from build123d import *

# Parameters (mm, degrees)
F0_W      = 35
F0_H      = 35
F1_DEPTH  = 40
F2_R      = 2.5
F3_DEPTH  = 20
F5_DEPTH  = 4.4
F6_R      = 4.25
F7_DEPTH  = 21
F8_R      = 2.5
F9_DEPTH  = 14.6
F11_DEPTH = 1.9
F12_R     = 0.5
F13_DEPTH = 4


with BuildPart() as f1:
    # F0 (on Top) → F1 (new body)
    with BuildSketch(Plane.XY):
        Rectangle(F0_W, F0_H)
    extrude(amount=F1_DEPTH)

    # F2 (on face) → F3 (cut)
    with BuildSketch(Plane(origin=(0, 0, 0), x_dir=(1, 0, 0), z_dir=(0, 0, -1))):
        with Locations((-10, 0)):
            Circle(F2_R)
        with Locations((10, 0)):
            Circle(F2_R)
    extrude(amount=-F3_DEPTH, mode=Mode.SUBTRACT)

    # F4 (on face) → F5 (cut)
    with BuildSketch(Plane.XY.offset(40)):
        Polygon((-17.5, -17.5), (17.5, -17.5), (17.5, -2.5), (3.35, -2.5), (3.35, 17.5), (-3.35, 17.5), (-3.35, -2.5), (-17.5, -2.5), align=None)
    extrude(amount=-F5_DEPTH, mode=Mode.SUBTRACT)

    # F6 (on face) → F7 (cut)
    with BuildSketch(Plane(origin=(0, 0, 0), x_dir=(1, 0, 0), z_dir=(0, 0, -1))):
        with Locations((0, -5.05)):
            Circle(F6_R)
    extrude(amount=-F7_DEPTH, mode=Mode.SUBTRACT)

    # F8 (on face) → F9 (cut, through all)
    with BuildSketch(Plane(origin=(0, 0, 21), x_dir=(1, 0, 0), z_dir=(0, 0, -1))):
        with Locations((0, -5.05)):
            Circle(F8_R)
    extrude(amount=-F9_DEPTH, mode=Mode.SUBTRACT)

    # F10 (on face) → F11 (cut)
    with BuildSketch(Plane.XY.offset(35.6)):
        Polygon((-5, -17.5), (5, -17.5), (5, -10.5), (1.575, -10.5), (1.575, -2.65), (-1.575, -2.65), (-1.575, -10.5), (-5, -10.5), align=None)
    extrude(amount=-F11_DEPTH, mode=Mode.SUBTRACT)

    # F12 (on face) → F13 (cut)
    with BuildSketch(Plane.XY.offset(35.6)):
        with Locations((-2.025, -9)):
            Circle(F12_R)
        with Locations((-2.025, -4)):
            Circle(F12_R)
        with Locations((2.025, -9)):
            Circle(F12_R)
        with Locations((2.025, -4)):
            Circle(F12_R)
        with Locations((-0.975, -2.2)):
            Circle(F12_R)
        with Locations((0.975, -2.2)):
            Circle(F12_R)
    extrude(amount=-F13_DEPTH, mode=Mode.SUBTRACT)


solid = f1.part
CAD build for the part. Positions are in the model's coordinates, mm. A direction names the side the tool comes from. Give positions to 0.01 mm unless a question says otherwise; leave off trailing zeros. Write each loop counter-clockwise with the first axis right and the second up, starting at its lowest first coordinate (ties: lowest second). Pieces come first, ordered by that corner, then holes. Notation, with made-up numbers: M 13,68 L 52,68 A26 cw 52,106 Z; hole C 21,69.25 d5. An arc over 180 degrees is marked long. Put each result on its own line as item: value. Start each with the question number.
(1) Band-saw the part on D-D, the plane y = 5.05. Write the cut outline in (x, z), and give its area (3 significant figures).
(2) Band-saw the part on B-B, the plane z = 35. Write the cut outline in (x, y) (3 decimals).
(3) Band-saw the part on C-C, the plane x = -10. Write the cut outline in (y, z), and give its area (3 significant figures).
(4) Which spindle directions (+Z, -Z, +X, -X, +Y, -Y) get a long thin tool onto all of the face, cutting with end or side? Do faces 4 (the face through (10, 0, 20)), 5 (the face through (1.575, -3, 35)), 6 (the face through (-2.525, -3.978, 33.628)), 7 (the face through (3.35, 7, 38)), 8 (the face through (0, 0, 0)). Say none if no direction does.
(5) Band-saw the part on A-A, the plane y = -13. Write the cut outline in (x, z).
(6) Mould opens along Y. For faces 1 (the face through (10, 8, 40)), 2 (the face through (3, -10.5, 35)), 3 (the face through (2, -4, 31.6)) say: +Y half, -Y half, draft (parallel to the pull), parting line (faces both ways), or undercut.
(7) Flat gauge pins, fed straight in: pin 1 Ø1.1 at (x, y) = (2, -9) entering from +Z; pin 2 Ø3.5 at (x, z) = (-9, 37.5) entering from -Y; pin 3 Ø4 at (x, y) = (-10, 0) entering from -Z; pin 4 Ø4 at (x, y) = (13, 4) entering from -Z. Where does each tip first touch, or does it go through?
(8) Probe L1, parallel to X at y = 0, z = 15; L2, parallel to X at y = 5.05, z = 27. List the from-to ranges inside material, lowest first.
Response values:
1. outline: M -17.5,0 L -4.25,0 L -4.25,21 L -2.5,21 L -2.5,35.6 L -3.35,35.6 L -3.35,40 L -17.5,40 Z; M 2.5,21 L 4.25,21 L 4.25,0 L 17.5,0 L 17.5,40 L 3.35,40 L 3.35,35.6 L 2.5,35.6 Z
1. area: 1,120 mm2
2. outline: M -17.5,-17.5 L -5,-17.5 L -5,-10.5 L -1.575,-10.5 L -1.575,-9.218 A0.5 cw long -1.575,-8.782 L -1.575,-4.218 A0.5 cw long -1.575,-3.782 L -1.575,-2.65 L -1.193,-2.65 A0.5 cw long -0.757,-2.65 L 0.757,-2.65 A0.5 cw long 1.193,-2.65 L 1.575,-2.65 L 1.575,-3.782 A0.5 cw long 1.575,-4.218 L 1.575,-8.782 A0.5 cw long 1.575,-9.218 L 1.575,-10.5 L 5,-10.5 L 5,-17.5 L 17.5,-17.5 L 17.5,17.5 L -17.5,17.5 Z; hole C 0,5.05 d5
3. outline: M -17.5,0 L -2.5,0 L -2.5,20 L 2.5,20 L 2.5,0 L 17.5,0 L 17.5,40 L -2.5,40 L -2.5,35.6 L -17.5,35.6 Z
3. area: 1,230 mm2
4. face 4: -Z
4. face 5: +Z, -Y
4. face 6: +Z
4. face 7: +Z, +Y, -Y
4. face 8: -Z, +X, -X, +Y, -Y
5. outline: M -17.5,0 L 17.5,0 L 17.5,35.6 L 5,35.6 L 5,33.7 L -5,33.7 L -5,35.6 L -17.5,35.6 Z
6. face 1: draft
6. face 2: -Y half
6. face 3: undercut
7. pin 1: stops at z = 35.6
7. pin 2: stops at y = -2.5
7. pin 3: stops at z = 20
7. pin 4: stops at z = 0
8. L1: x = -17.5 to -12.5, -7.5 to 7.5, 12.5 to 17.5
8. L2: x = -17.5 to -2.5, 2.5 to 17.5
